The drawing under review shows one solid part. Ordinate dimensions are in mm from its lowest x, y, z. A direction names the side the tool comes from. Coordinates: 2 decimals unless noted, no trailing zeros. Loops run counter-clockwise (first coordinate to the right, second up) from the corner with the lowest first, then second, coordinate; pieces in that order, holes last. Notation, with made-up numbers: (40, 1.25) -> (82, 1.25) arc R8 cw to (82, 5.25) -> close; hole circle Ø11 at (11, 76.5). An arc over 180 degrees is marked (long way). Use a Markdown table: item, result.
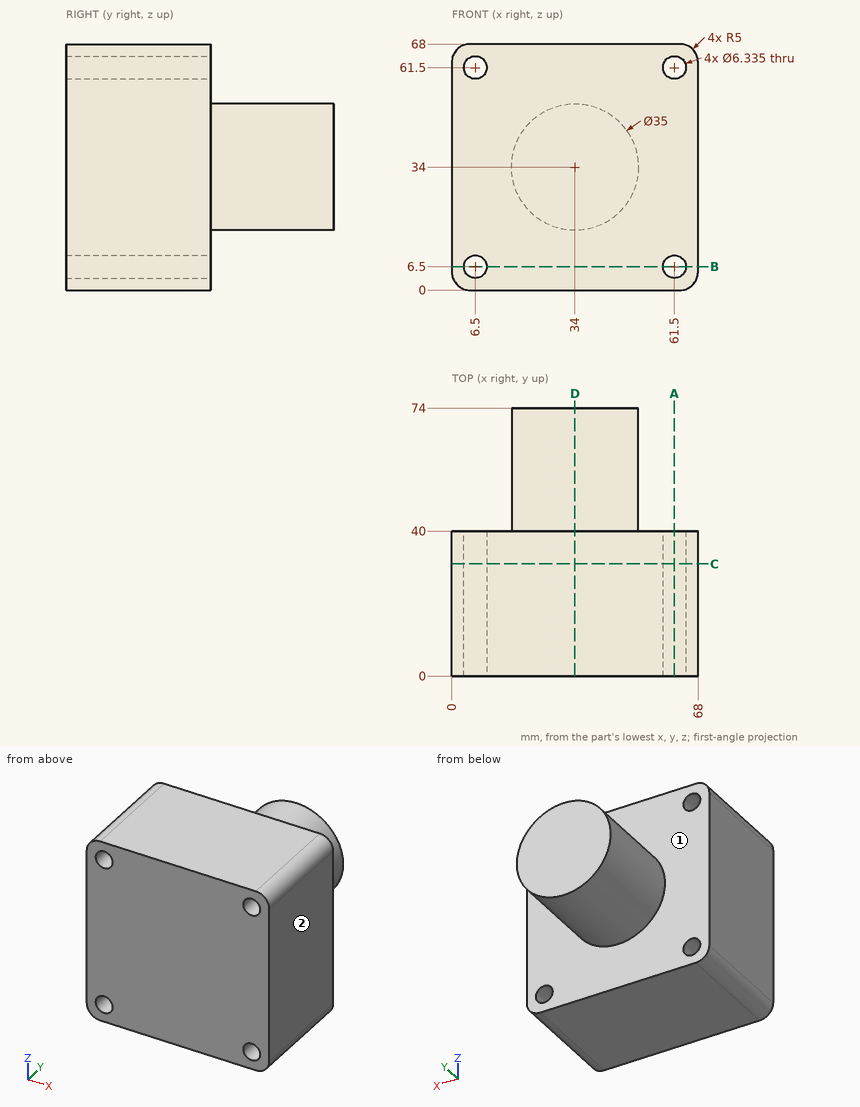
(1) Take a section at D-D on x = 34. Write out the cut boundary in (y, z), plus the area to 3 significant figures.
Found:
| item | result |
|---|---|
| outline | (0, 0) -> (40, 0) -> (40, 16.5) -> (74, 16.5) -> (74, 51.5) -> (40, 51.5) -> (40, 68) -> (0, 68) -> close |
| area | 3,910 mm^2 |
(2) For the marked faces 1 and 2, list the 3-axis set-ups (+Z, -Z, +X, -X, +Y, -Y) from which the entire face can be reached by the end or side of a thin tool; tool diameter is ignored.
Found:
| item | result |
|---|---|
| face 1 | +Y |
| face 2 | +Z, -Z, +X, +Y, -Y |
(3) Take a section at B-B on z = 6.5. Write out the cut boundary in (x, y), plus the area to 3 significant figures.
Found:
| item | result |
|---|---|
| outline | (0, 0) -> (3.33, 0) -> (3.33, 40) -> (0, 40) -> close; (9.67, 0) -> (58.33, 0) -> (58.33, 40) -> (9.67, 40) -> close; (64.67, 0) -> (68, 0) -> (68, 40) -> (64.67, 40) -> close |
| area | 2,210 mm^2 |
(4) For line 1 along Z through (x, y) = (6.5, 24); line 2 along Z through (x, y) = (6, 31), list the stretches that pass through material, from the lowest coordinate up.
Found:
| item | result |
|---|---|
| line 1 | z = 0 to 3.33, 9.67 to 58.33, 64.67 to 68 |
| line 2 | z = 0 to 3.37, 9.63 to 58.37, 64.63 to 68 |
(5) Take a section at A-A on x = 61.5. Write out the cut boundary in (y, z).
Found:
| item | result |
|---|---|
| outline | (0, 0) -> (40, 0) -> (40, 3.33) -> (0, 3.33) -> close; (0, 9.67) -> (40, 9.67) -> (40, 58.33) -> (0, 58.33) -> close; (0, 64.67) -> (40, 64.67) -> (40, 68) -> (0, 68) -> close |
(6) Take a section at C-C on y = 31. Write out the cut boundary in (x, z) (1 decimal).
Found:
| item | result |
|---|---|
| outline | (0, 5) arc R5 ccw to (5, 0) -> (63, 0) arc R5 ccw to (68, 5) -> (68, 63) arc R5 ccw to (63, 68) -> (5, 68) arc R5 ccw to (0, 63) -> close; hole circle Ø6.3 at (6.5, 6.5); hole circle Ø6.3 at (6.5, 61.5); hole circle Ø6.3 at (61.5, 6.5); hole circle Ø6.3 at (61.5, 61.5) |
(7) For pin 1 Ø12 at (y, z) = (60, 7) entering from -X; pin 2 Ø7.5 at (x, z) = (61.5, 61.5) entering from +Y, all flat-tipped, find the tip position at first contact; note any pin that passes through.
Found:
| item | result |
|---|---|
| pin 1 | passes through |
| pin 2 | stops at y = 40 |
